Verification items for the finished model (mm, model axes). A direction names the side the tool comes from. Give positions to 0.01 mm unless a question says otherwise; leave off trailing zeros. Loops run counter-clockwise (first coordinate to the right, second up) from the corner with the lowest first, then second, coordinate; pieces in that order, holes last. Notation, with made-up numbers: (47, 18) -> (93, 18) arc R19 cw to (93, 52) -> close; hole circle Ø6 at (1, -11.5). An arc over 180 degrees is marked (long way). Answer in a Markdown table with one row per item. Add a question column.
Q1. Gauge pin test, flat ends, axial feed: P1, Ø2, axis at x = -3, z = 3, coming from the -Y side; P2, Ø1, axis at x = 6, z = 0, coming from the +Y side; P3, Ø6, axis at x = -4.5, z = 2.5, coming from the +Y side. Record the tip position at first contact, or that the pin passes through.
Q2. Release check for a two-part mould opening along X. For faces 4 (the face through (0, 8.2, 5.29)), 5 (the face through (-4, -6, -0.69)), 6 (the face through (-8.881, -8.144, -0.045)) record: pulls with the +X half, pulls with the -X half, needs draft (parallel to the pull), parting line crosses it, or undercut.
Q3. Section check A-A on x = 0. Enter the section's corners in (y, z), and give its area (3 significant figures).
Q4. Set-up check for faces 1 (the face through (-1.47, 6.64, -0.01)), 2 (the face through (-1.73, 7.81, 2.96)), 3 (the face through (-1.73, -7.81, -2.96)): record each of +Z, -Z, +X, -X, +Y, -Y from which the full face is reachable in a straight line by a thin tool's end or side.
Q5. Material ranges on probe 1 along X at (y, z) = (-2.5, 3.5); probe 2 along Y at (x, z) = (5.5, -0.5); probe 3 along Y at (x, z) = (0, 4), recorded low to high.
Q6. Section check C-C on z = 2.75. Enter the section's corners in (x, y).
Autodesk Inventor part; units mm, degrees
ref_plane "YZ Plane" through (0, 0, 0) normal (1, 0, 0) x (0, 1, 0)
ref_plane "XZ Plane" through (0, 0, 0) normal (0, 1, 0) x (-1, 0, 0)
ref_plane "XY Plane" through (0, 0, 0) normal (0, 0, 1) x (1, 0, 0)
sketch "Sketch1" plane through (0, 0, 0) normal (0, 0, 1) x (1, 0, 0)
  circle A0 centre (0, 0) radius 6.8
  circle A1 centre (0, 0) radius 12.05
  dimension "d10" = 13.6
  dimension "d11" = 24.1
extrude "Extrusion3" add sketch "Sketch1" along normal mid plane 1.38
sketch "Sketch2" plane through (0, 0, 0) normal (0, 0, 1) x (1, 0, 0)
  circle A0 centre (0, 0) radius 12.05
  circle A1 centre (0, 0) radius 8
  dimension "d14" = 24.1
  dimension "d15" = 16
extrude "Extrusion4" add sketch "Sketch2" along normal mid plane 10.58
chamfer "Chamfer2" distance 2.05 angle 45 2 edges at (-12.05, 0, 5.29) (-12.05, 0, -5.29)
properties part number "Rollers" material "Acetal Resin, Black"
Taken from the geometry:
| question | item | result |
|---|---|---|
| 1 | P1 | stops at y = -11.88 |
| 1 | P2 | stops at y = 10.72 |
| 1 | P3 | stops at y = 11.96 |
| 2 | face 4 | needs draft |
| 2 | face 5 | undercut |
| 2 | face 6 | parting line crosses it |
| 3 | outline | (-12.05, -3.24) -> (-10, -5.29) -> (-8, -5.29) -> (-8, -0.69) -> (-6.8, -0.69) -> (-6.8, 0.69) -> (-8, 0.69) -> (-8, 5.29) -> (-10, 5.29) -> (-12.05, 3.24) -> close; (6.8, -0.69) -> (8, -0.69) -> (8, -5.29) -> (10, -5.29) -> (12.05, -3.24) -> (12.05, 3.24) -> (10, 5.29) -> (8, 5.29) -> (8, 0.69) -> (6.8, 0.69) -> close |
| 3 | area | 80.6 mm² |
| 4 | face 1 | +Z, -Z |
| 4 | face 2 | +Z |
| 4 | face 3 | -Z |
| 5 | probe 1 | x = -11.52 to -7.6, 7.6 to 11.52 |
| 5 | probe 2 | y = -10.72 to -4, 4 to 10.72 |
| 5 | probe 3 | y = -11.29 to -8, 8 to 11.29 |
| 6 | outline | circle Ø24.1 at (0, 0); hole circle Ø16 at (0, 0) |
